For this review, take the finished solid that the model builds, in its own axes (mm). Face numbers are marked on the shaded views. A direction names the side the tool comes from. Coordinates: 2 decimals unless noted, no trailing zeros. Loops run counter-clockwise (first coordinate to the right, second up) from the corner with the lowest first, then second, coordinate; pieces in that order, holes last. Notation, with made-up numbers: (72.5, -2.75) -> (80.5, -2.75) arc R17 ccw to (80.5, 22.25) -> close; hole circle Ø7 at (0.25, -36). An arc over 180 degrees is marked (long way). Use a Markdown table: item, result.
from build123d import *

# Parameters (mm, degrees)
F0_R     = 6
F1_DEPTH = 100
F3_DEPTH = 100


with BuildPart() as f1:
    # F0 (on Top) → F1 (new body)
    with BuildSketch(Plane.XY):
        Circle(F0_R)
    extrude(amount=F1_DEPTH)

    # F2 (on face) → F3 (join)
    with BuildSketch(Plane(origin=(0, 0, 0), x_dir=(1, 0, 0), z_dir=(0, 0, -1))):
        with BuildLine():
            ThreePointArc((0, -6), (-4.2426406871, -4.2426406871), (-6, 0))
            Line((-6, 0), (-10, 0))
            Line((-10, 0), (-10, -5))
            ThreePointArc((-10, -5), (-8.5355339059, -8.5355339059), (-5, -10))
            Line((-5, -10), (0, -10))
            Line((0, -10), (0, -6))
        make_face()
        with BuildLine():
            Line((-10, 0), (-6, 0))
            ThreePointArc((-6, 0), (-4.2426406871, 4.2426406871), (0, 6))
            Line((0, 6), (0, 10))
            Line((0, 10), (-5, 10))
            ThreePointArc((-5, 10), (-8.5355339059, 8.5355339059), (-10, 5))
            Line((-10, 5), (-10, 0))
        make_face()
        with BuildLine():
            ThreePointArc((0, 6), (-4.2426406871, 4.2426406871), (-6, 0))
            ThreePointArc((-6, 0), (-4.2426406871, -4.2426406871), (0, -6))
            ThreePointArc((0, -6), (4.2426406871, -4.2426406871), (6, 0))
            ThreePointArc((6, 0), (4.2426406871, 4.2426406871), (0, 6))
        make_face()
        with BuildLine():
            Line((0, 10), (0, 6))
            ThreePointArc((0, 6), (4.2426406871, 4.2426406871), (6, 0))
            Line((6, 0), (10, 0))
            Line((10, 0), (10, 5))
            ThreePointArc((10, 5), (8.5355339059, 8.5355339059), (5, 10))
            Line((5, 10), (0, 10))
        make_face()
        with BuildLine():
            ThreePointArc((6, 0), (4.2426406871, -4.2426406871), (0, -6))
            Line((0, -6), (0, -10))
            Line((0, -10), (5, -10))
            ThreePointArc((5, -10), (8.5355339059, -8.5355339059), (10, -5))
            Line((10, -5), (10, 0))
            Line((10, 0), (6, 0))
        make_face()
    extrude(amount=F3_DEPTH)


solid = f1.part
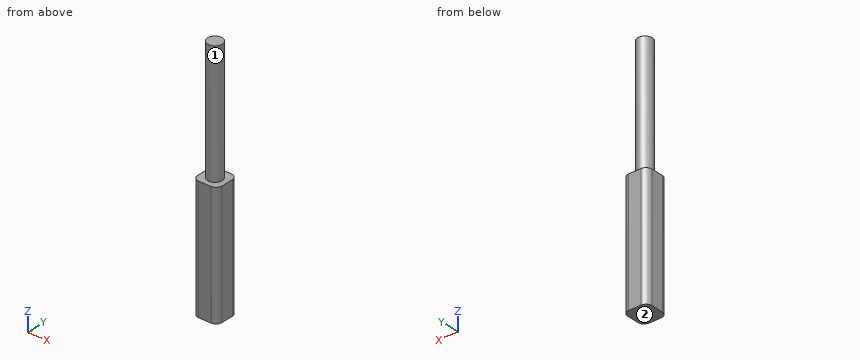
(1) For pin 1 Ø5 at (y, z) = (3.5, 67) entering from +X; pin 2 Ø1.5 at (y, z) = (-1.5, 7) entering from -X; pin 3 Ø3 at (y, z) = (-1.5, 30) entering from +X; pin 4 Ø8 at (x, y) = (5.5, 3) entering from +Z, all flat-tipped, find the tip position at first contact; note any pin that passes through.
Found:
| item | result |
|---|---|
| pin 1 | stops at x = 5.92 |
| pin 2 | stops at x = -5.95 |
| pin 3 | stops at x = 6 |
| pin 4 | stops at z = 100 |
(2) Take a section at A-A on x = 0. Write out the cut boundary in (y, z).
Found:
| item | result |
|---|---|
| outline | (-10, -100) -> (10, -100) -> (10, 0) -> (6, 0) -> (6, 100) -> (-6, 100) -> (-6, 0) -> (-10, 0) -> close |
(3) Take a section at C-C on z = 33.5. Write out the cut boundary in (x, y).
Found:
| item | result |
|---|---|
| outline | circle Ø12 at (0, 0) |
(4) Take a section at D-D on x = -8. Write out the cut boundary in (y, z), plus the area to 3 significant figures.
Found:
| item | result |
|---|---|
| outline | (-9, -100) -> (9, -100) -> (9, 0) -> (-9, 0) -> close |
| area | 1,800 mm^2 |
(5) For line 1 along Z through (x, y) = (0, 7); line 2 along X through (y, z) = (5.25, -16); line 3 along Y through (x, z) = (0.5, 53), list the stretches that pass through material, from the lowest coordinate up.
Found:
| item | result |
|---|---|
| line 1 | z = -100 to 0 |
| line 2 | x = -9.99 to 9.99 |
| line 3 | y = -5.98 to 5.98 |
(6) For the marked faces 1 and 2, list the 3-axis set-ups (+Z, -Z, +X, -X, +Y, -Y) from which the entire face can be reached by the end or side of a thin tool; tool diameter is ignored.
Found:
| item | result |
|---|---|
| face 1 | +Z |
| face 2 | -Z, +X, -X, +Y, -Y |
